Autodesk Inventor part; units mm, degrees
ref_plane "YZ Plane" through (0, 0, 0) normal (1, 0, 0) x (0, 1, 0)
ref_plane "XZ Plane" through (0, 0, 0) normal (0, 1, 0) x (-1, 0, 0)
ref_plane "XY Plane" through (0, 0, 0) normal (0, 0, 1) x (1, 0, 0)
sketch "Skizze1" plane through (0, 0, 0) normal (0, 0, 1) x (1, 0, 0)
  circle A0 centre (0, 0) radius 34.775
  dimension "d0" = 69.55
extrude "Extrusion1" add sketch "Skizze1" along normal blind 5
sketch "Skizze2" plane through (0, 0, 5) normal (0, 0, 1) x (1, 0, 0)
  circle A0 centre (0, 0) radius 32.54
  dimension "d3" = 65.08
extrude "Extrusion2" cut sketch "Skizze2" against normal blind 3
sketch "Skizze3" plane through (0, 0, 0) normal (0, 0, -1) x (-1, 0, 0)
  circle A0 centre (0, 0) radius 7.56
  dimension "d6" = 15.12
extrude "Extrusion3" cut sketch "Skizze3" against normal through all
sketch "Skizze4" plane through (0, 0, 5) normal (0, 0, 1) x (1, 0, 0)
  line L0 (-8, -42.775) -> (8, -42.775)
  line L1 (8, -42.775) -> (8, -26.775)
  line L2 (8, -26.775) -> (-8, -26.775)
  line L3 (-8, -26.775) -> (-8, -42.775)
  circle A0 centre (0, 0) radius 34.775
  line L4 (-8, -42.775) -> (8, -26.775) construction
  line L5 (8, -42.775) -> (-8, -26.775) construction
  point P0 (0, -34.775)
  dimension "d9" = 16
  dimension "d10" = 16
extrude "Extrusion4" cut sketch "Skizze4" against normal up to surface (3 mm away) contours L3 A0 L1 L0 | L3 L2 L1 A0 picked at (0.896, -29.407)
properties part number "2024_08_28_Holder_disk_GCvial"
Geometry: final body of the model. Coordinates: model frame, mm. A direction names the side the tool comes from. Coordinates: 2 decimals unless noted, no trailing zeros. Order: outer loops, then holes, each group sorted by start corner. A loop starts at its lowest first (then second) coordinate and runs counter-clockwise, first axis right, second up.
1) Section C-C (y = -25.5). Return loops of the section in (x, z).
Result sheet:
outline: (-23.64, 0) - (23.64, 0) - (23.64, 5) - (20.21, 5) - (20.21, 2) - (-20.21, 2) - (-20.21, 5) - (-23.64, 5) - close
2) Section B-B (y = 0). Return loops of the section in (x, z) (3 decimals).
Result sheet:
outline: (-34.775, 0) - (-7.56, 0) - (-7.56, 2) - (-32.54, 2) - (-32.54, 5) - (-34.775, 5) - close; (7.56, 0) - (34.775, 0) - (34.775, 5) - (32.54, 5) - (32.54, 2) - (7.56, 2) - close
3) Section D-D (x = 24.5). Return loops of the section in (y, z).
Result sheet:
outline: (-24.68, 0) - (24.68, 0) - (24.68, 5) - (21.41, 5) - (21.41, 2) - (-21.41, 2) - (-21.41, 5) - (-24.68, 5) - close
4) Ray query, probe 1 along X at (y, z) = (0, 3.6) (3 decimals); probe 2 along Y at (x, z) = (0, 1.5) (3 decimals); probe 3 along Z at (x, y) = (8, -5.5). Return the intervals inside material, ascending.
Result sheet:
probe 1: x = -34.775 to -32.54, 32.54 to 34.775
probe 2: y = -34.775 to -7.56, 7.56 to 34.775
probe 3: z = 0 to 2
5) Draft query along X for faces 4 (the flat face through (-8, -33, 4)), 5 (the flat face through (10.1, 31.1, 5)), 6 (the cylindrical face through (-7.539, 33.948, 2.465)). Return one class per face: released by +X, released by -X, zero draft, split by the parting line, or undercut.
Result sheet:
face 4: undercut
face 5: zero draft
face 6: split by the parting line
6) Section A-A (x = 0). Return loops of the section in (y, z) (3 decimals).
Result sheet:
outline: (-34.775, 0) - (-7.56, 0) - (-7.56, 2) - (-34.775, 2) - close; (7.56, 0) - (34.775, 0) - (34.775, 5) - (32.54, 5) - (32.54, 2) - (7.56, 2) - close
7) First-contact query: P1, Ø5, axis at x = 6.5, y = -16, coming from the +Z side; P2, Ø0.7, axis at y = -32.5, z = 3.5, coming from the -X side; P3, Ø5, axis at x = 2.5, y = -19, coming from the -Z side; P4, Ø1.8, axis at y = -32.5, z = 4, coming from the +X side. Flat tips, straight axial feed; report the tip coordinate or a pass-through.
Result sheet:
P1: stops at z = 2
P2: stops at x = -13.25
P3: stops at z = 0
P4: stops at x = 14.52
8) Set-up query: faces 1 (the flat face through (8, -33, 4)), 2 (the flat face through (0, 8, 0)), 3 (the cylindrical face through (1.318, 32.513, 3.521)). Return all of +Z, -Z, +X, -X, +Y, -Y with unobstructed straight access to the full face (end or side cutting, diameter ignored); none if empty.
Result sheet:
face 1: +Z, -Y
face 2: -Z, +X, -X, +Y, -Y
face 3: +Z
